from build123d import *

# Parameters (mm, degrees)
SKETCH3_R   = 20.6375
SKETCH3_R_2 = 13.3223


with BuildPart() as part:
    # Sketch1 → Revolve1 (revolve)
    with BuildSketch(Plane.XY, mode=Mode.PRIVATE) as revolve1_sk:
        Polygon((-42.06875, -20.6375), (-17.4625, -20.6375), (-17.4625, -16.637), (-42.06875, -16.8275), align=None)
    revolve(revolve1_sk.sketch.rotate(Axis((-42.06875, 0, 0), (1, 0, 0)), 270), axis=Axis((-42.06875, 0, 0), (1, 0, 0)))


with BuildPart() as body_2:
    # Sketch2 → Revolve2 (revolve)
    with BuildSketch(Plane.XY, mode=Mode.PRIVATE) as revolve2_sk:
        Polygon((16.8275, 42.06875), (16.637, 17.4625), (20.6375, 17.4625), (20.6375, 42.06875), align=None)
    revolve(revolve2_sk.sketch.rotate(Axis((0, 0, 0), (0, 1, 0)), 90), axis=Axis((0, 0, 0), (0, 1, 0)))


with BuildPart() as sweep1_tool:
    # Sweep1: sweep along a path in Sketch4
    with BuildLine(Plane.XY) as sweep1_path:
        ThreePointArc((-17.4625, 0), (-5.114648, 5.114648), (0, 17.4625))
    # Sketch3 → Sweep1 (sweep)
    with BuildSketch(Plane(origin=(-17.4625, 0, 0), x_dir=(0, 0, -1), z_dir=(1, 0, 0))):
        Circle(SKETCH3_R)
        Circle(SKETCH3_R_2, mode=Mode.SUBTRACT)
    sweep(path=sweep1_path.line)


with BuildPart() as part_1:
    add(part.part)


with BuildPart() as part_2:
    # Sweep1: joined with sweep1_tool
    add(part_1.part.fuse(sweep1_tool.part, body_2.part, tol=0.00001))


solid = part_2.part
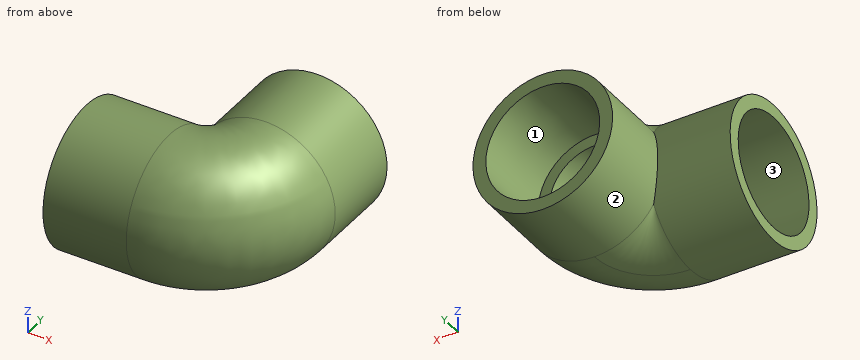
Design review of the part built by this model. Coordinates are the model's own, in mm. Face numbers are marked on the shaded views. Give positions to 0.01 mm unless a question says otherwise; leave off trailing zeros. Write each loop counter-clockwise with the first axis right and the second up, starting at its lowest first coordinate (ties: lowest second). Pieces come first, ordered by that corner, then holes. Notation, with made-up numbers: M 73.5,73 L 104.5,73 A29 cw 104.5,112 Z; hole C -14.75,66.25 d2. An arc over 180 degrees is marked long. Answer as a JSON object with one key per item and string values. Group by question number.
1) For line 1 along Y through (x, z) = (-28, -4); line 2 along Y through (x, z) = (-35, 7.5); line 3 along Z through (x, y) = (-25.5, -14.5), list the stretches that pass through material, from the lowest coordinate up.
2) Clearance check with flat-ended pins moving along their axes: pin 1 Ø3 at (x, y) = (-20.5, 28.5) entering from +Z; pin 2 Ø1 at (x, z) = (4, 11.5) entering from -Y; pin 3 Ø8 at (x, z) = (-26.5, 2) entering from -Y. State where each tip first meets the part, or that it passes through.
3) Mouldability with a two-part tool opening along X and no side actions: class the marked faces 1, 2 and 3 as released by +X, released by -X, zero draft, split by the parting line, or undercut.
4) We need section A-A (x = -34). Give the boundary of the cut face in (y, z) (1 decimal), and give its area (3 significant figures).
Answer key:
{
 "1": {"line 1": "y = -20.25 to -16.23, 16.23 to 20.25", "line 2": "y = -19.23 to -15, 15 to 19.23", "line 3": "z = -14.69 to -8.28, 8.28 to 14.69"},
 "2": {"pin 1": "stops at z = 8.06", "pin 2": "stops at y = -10.24", "pin 3": "stops at y = -20.64"},
 "3": {"face 1": "undercut", "face 2": "split by the parting line", "face 3": "released by -X"},
 "4": {"outline": "C 0,0 d41.3; hole C 0,0 d33.5", "area": "455 mm²"}
}
